Source: CAD feature listing. Evaluate the final solid. Frame: model axes, mm. Face numbers are marked on the shaded views. A direction names the side the tool comes from. Coordinates: 2 decimals unless noted, no trailing zeros. Order: outer loops, then holes, each group sorted by start corner. A loop starts at its lowest first (then second) coordinate and runs counter-clockwise, first axis right, second up. Notation, with made-up numbers: (29.25, 48.5) - (54.25, 48.5) arc R8 ccw to (54.25, 63.5) - close; hole circle Ø1 at (40, 51.5). An arc over 180 degrees is marked (long way). One line per question, with ' | ' between items.
from build123d import *

# Parameters (mm, degrees)
ESQUISSE2_W             = 8.320302529
ESQUISSE2_H             = 23.371875391
ESQUISSE2_W_2           = 7.922092332
ENL_V_MAT_EXTRU_1_DEPTH = 32
ENL_V_START             = -2
ENL_V_MAT_EXTRU_2_DEPTH = 2
ESQUISSE4_R             = 1
ENL_V_MAT_EXTRU_3_DEPTH = 4


with BuildPart() as part:
    # Esquisse1 → Révolution1 (revolve)
    with BuildSketch(Plane.XY, mode=Mode.PRIVATE) as r_volution1_sk:
        Polygon((-13.035736805, 0), (-13.035736805, -2), (-3, -2), (-3, -4), (-2, -4), (-2, -7), (0, -7), (0, -11), (21.7, -11), (21.7, -10.25), (53.7, -10.25), (53.7, -3), (55.7, -3), (55.7, 0), align=None)
    revolve(r_volution1_sk.sketch.rotate(Axis((38.703399471, 0, 0), (-1, 0, 0)), 270), axis=Axis((38.703399471, 0, 0), (-1, 0, 0)))

    # Esquisse2 → Enlèv. mat.-Extru.1 (cut)
    with BuildSketch(Plane(origin=(53.7, 0, 0), x_dir=(0, 0, -1), z_dir=(1, 0, 0))):
        with Locations((-11.860151265, -0.490104857)):
            Rectangle(ESQUISSE2_W, ESQUISSE2_H)
        with Locations((11.661046166, -0.490104857)):
            Rectangle(ESQUISSE2_W_2, ESQUISSE2_H)
    extrude(amount=-ENL_V_MAT_EXTRU_1_DEPTH, mode=Mode.SUBTRACT)

    # Esquisse3 → Enlèv. mat.-Extru.2 (cut)
    with BuildSketch(Plane.ZY.offset(2).offset(ENL_V_START)):
        with BuildLine():
            Line((6.792150444, 1.69313093), (1.69313093, 6.792150444))
            ThreePointArc((1.69313093, 6.792150444), (4.949747468, 4.949747468), (6.792150444, 1.69313093))
        make_face()
        with BuildLine():
            Line((-6.792150444, -1.69313093), (-1.69313093, -6.792150444))
            ThreePointArc((-1.69313093, -6.792150444), (-4.949747468, -4.949747468), (-6.792150444, -1.69313093))
        make_face()
    extrude(amount=ENL_V_MAT_EXTRU_2_DEPTH, mode=Mode.SUBTRACT)

    # Esquisse4 → Enlèv. mat.-Extru.3 (cut)
    with BuildSketch(Plane.ZY):
        with Locations((0, 9)):
            Circle(ESQUISSE4_R)
        with Locations((-9, 0)):
            Circle(ESQUISSE4_R)
        with Locations((0, -9)):
            Circle(ESQUISSE4_R)
        with Locations((9, 0)):
            Circle(ESQUISSE4_R)
    extrude(amount=-ENL_V_MAT_EXTRU_3_DEPTH, mode=Mode.SUBTRACT)


solid = part.part
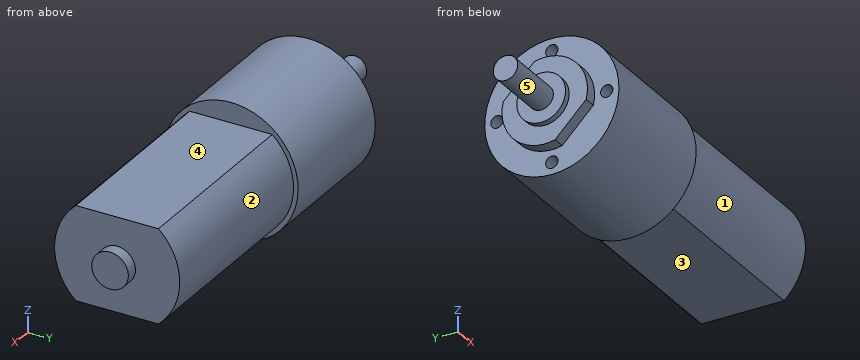
(1) Pin query (flat end, axial travel): P1, Ø12, axis at x = 36.5, y = 8, coming from the +Z side; P2, Ø11, axis at x = 36, y = -1, coming from the -Z side; P3, Ø1.6, axis at y = -9.5, z = -0.5, coming from the -X side. Return the tip coordinate at first contact, or that it passes through.
Taken from the geometry:
P1: stops at z = 7.7 | P2: stops at z = -7.7 | P3: stops at x = 0
(2) Set-up query: the marked faces 1, 2, 3, 4 and 5. Return all of +Z, -Z, +X, -X, +Y, -Y with unobstructed straight access to the full face (end or side cutting, diameter ignored); none if empty.
Taken from the geometry:
face 1: +X, -Y | face 2: +X, +Y | face 3: -Z, +X, +Y, -Y | face 4: +Z, +X, +Y, -Y | face 5: -X
(3) Material intervals for L1, parallel to Y at x = 2.75, z = 0; L2, parallel to X at y = 1.25, z = 4.75; L3, parallel to X at y = 5.5, z = -7.25, sorted ascending. Write a range as from..to.
Taken from the geometry:
L1: y = -11..-10, -8..8, 10..11 | L2: x = -2..53.7 | L3: x = 0..53.7
(4) Cut plane D-D (z = 9). Return the cut outline in (x, y), and give its area (3 significant figures).
Taken from the geometry:
outline: (0, -6.32) - (21.7, -6.32) - (21.7, 6.32) - (0, 6.32) - (0, 1) - (4, 1) - (4, -1) - (0, -1) - close | area: 266 mm²
(5) Cut plane C-C (x = 46.5). Return the cut outline in (y, z).
Taken from the geometry:
outline: (-6.77, -7.7) - (6.77, -7.7) arc R10.25 ccw to (6.77, 7.7) - (-6.77, 7.7) arc R10.25 ccw to start
